```python
from build123d import *

# Parameters (mm, degrees)
SKETCH1_W                                       = 200
SKETCH1_H                                       = 320
BOSS_EXTRUDE1_DEPTH                             = 3.175
CSK_FOR_M3_FLAT_HEAD_MACHINE_SCREW1_D           = 3.4
CSK_FOR_M3_FLAT_HEAD_MACHINE_SCREW1_CSINK_D     = 6.3
CSK_FOR_M3_FLAT_HEAD_MACHINE_SCREW1_CSINK_ANGLE = 90
MIRROR2_COPY_1_D                                = 3.4
MIRROR2_COPY_1_CSINK_D                          = 6.3
MIRROR2_COPY_1_CSINK_ANGLE                      = 90
CSK_FOR_M4_FLAT_HEAD_MACHINE_SCREW1_AT_2_COUNT  = 2
CSK_FOR_M4_FLAT_HEAD_MACHINE_SCREW1_AT_2_PITCH  = 64.709214954
CSK_FOR_M4_FLAT_HEAD_MACHINE_SCREW1_AT_3_COUNT  = 2
CSK_FOR_M4_FLAT_HEAD_MACHINE_SCREW1_AT_3_PITCH  = 44.433123905
CSK_FOR_M4_FLAT_HEAD_MACHINE_SCREW1_AT_4_COUNT  = 2
CSK_FOR_M4_FLAT_HEAD_MACHINE_SCREW1_AT_4_PITCH  = 75.973301231
CSK_FOR_M4_FLAT_HEAD_MACHINE_SCREW1_AT_5_COUNT  = 2
CSK_FOR_M4_FLAT_HEAD_MACHINE_SCREW1_AT_5_PITCH  = 78.545162168
CSK_FOR_M4_FLAT_HEAD_MACHINE_SCREW1_AT_6_COUNT  = 2
CSK_FOR_M4_FLAT_HEAD_MACHINE_SCREW1_AT_6_PITCH  = 60.96
CSK_FOR_M4_FLAT_HEAD_MACHINE_SCREW1_AT_7_COUNT  = 2
CSK_FOR_M4_FLAT_HEAD_MACHINE_SCREW1_AT_7_PITCH  = 49.53
CSK_FOR_M4_FLAT_HEAD_MACHINE_SCREW1_AT_8_COUNT  = 2
CSK_FOR_M4_FLAT_HEAD_MACHINE_SCREW1_AT_8_PITCH  = 89.358393562
CSK_FOR_M4_FLAT_HEAD_MACHINE_SCREW1_AT_9_COUNT  = 2
CSK_FOR_M4_FLAT_HEAD_MACHINE_SCREW1_AT_9_PITCH  = 245.539452023
CSK_FOR_M4_FLAT_HEAD_MACHINE_SCREW1_AT_1_COUNT  = 2
CSK_FOR_M4_FLAT_HEAD_MACHINE_SCREW1_AT_1_PITCH  = 233.172012257
CSK_FOR_M4_FLAT_HEAD_MACHINE_SCREW1_2_COUNT     = 2
CSK_FOR_M4_FLAT_HEAD_MACHINE_SCREW1_2_PITCH     = 183.831254144
CSK_FOR_M4_FLAT_HEAD_MACHINE_SCREW1_3_COUNT     = 2
CSK_FOR_M4_FLAT_HEAD_MACHINE_SCREW1_3_PITCH     = 199.284633627
CSK_FOR_M4_FLAT_HEAD_MACHINE_SCREW1_4_COUNT     = 2
CSK_FOR_M4_FLAT_HEAD_MACHINE_SCREW1_4_PITCH     = 64.860029294
CSK_FOR_M4_FLAT_HEAD_MACHINE_SCREW1_5_COUNT     = 2
CSK_FOR_M4_FLAT_HEAD_MACHINE_SCREW1_5_PITCH     = 190.701291553
CSK_FOR_M4_FLAT_HEAD_MACHINE_SCREW1_6_COUNT     = 2
CSK_FOR_M4_FLAT_HEAD_MACHINE_SCREW1_6_PITCH     = 183.209354019
CSK_FOR_M4_FLAT_HEAD_MACHINE_SCREW1_7_COUNT     = 2
CSK_FOR_M4_FLAT_HEAD_MACHINE_SCREW1_7_PITCH     = 69.556924889
SKETCH8_R                                       = 19
CUT_EXTRUDE1_DEPTH                              = 4.175


with BuildPart() as part:
    # Sketch1 → Boss-Extrude1 (new body)
    with BuildSketch(Plane(origin=(0, 0, 0), x_dir=(1, 0, 0), z_dir=(0, 1, 0))):
        Rectangle(SKETCH1_W, SKETCH1_H)
    extrude(amount=BOSS_EXTRUDE1_DEPTH)

    # CSK for M3 Flat Head Machine Screw1 (through all)
    with Locations(Plane.XZ):
        with Locations((-95, 155), (-85, 155), (-95, 145), (-95, 135), (-95, 105), (-95, 95)):
            csk_for_m3_flat_head_machine_screw1 = CounterSinkHole(CSK_FOR_M3_FLAT_HEAD_MACHINE_SCREW1_D / 2, CSK_FOR_M3_FLAT_HEAD_MACHINE_SCREW1_CSINK_D / 2, counter_sink_angle=CSK_FOR_M3_FLAT_HEAD_MACHINE_SCREW1_CSINK_ANGLE)

    # Mirror1: CSK for M3 Flat Head Machine Screw1 across plane
    add(csk_for_m3_flat_head_machine_screw1.mirror(Plane(origin=(0, 0, 0), x_dir=(0, 0, 1), z_dir=(1, 0, 0))), mode=Mode.SUBTRACT)

    # Mirror2: CSK for M3 Flat Head Machine Screw1 across plane
    add(csk_for_m3_flat_head_machine_screw1.mirror(Plane.XY), mode=Mode.SUBTRACT)

    # Mirror2 copy 1 (through all)
    with Locations(Plane(origin=(0, 0, 0), x_dir=(-1, 0, 0), z_dir=(0, -1, 0))):
        with Locations((-95, 155), (-85, 155), (-95, 145), (-95, 135), (-95, 105), (-95, 95)):
            CounterSinkHole(MIRROR2_COPY_1_D / 2, MIRROR2_COPY_1_CSINK_D / 2, counter_sink_angle=MIRROR2_COPY_1_CSINK_ANGLE)

    # Sketch6 → CSK for M4 Flat Head Machine Screw1 (revolve, cut)
    with BuildSketch(Plane(origin=(-9.04, 0, 91.47), x_dir=(0, 0, -1), z_dir=(1, 0, 0))):
        Polygon((0, 0), (0, 3.175), (2.25, 3.175), (2.25, 2.45), (4.7, 0), align=None)
    csk_for_m4_flat_head_machine_screw1 = revolve(axis=Axis((-9.04, -6.35, 91.47), (0, 1, 0)), mode=Mode.SUBTRACT)

    # CSK for M4 Flat Head Machine Screw1 at 2: CSK for M4 Flat Head Machine Screw1 ×2
    with Locations(*[Vector(0.634221881, 0, 0.773151089) * (i * CSK_FOR_M4_FLAT_HEAD_MACHINE_SCREW1_AT_2_PITCH) for i in range(1, CSK_FOR_M4_FLAT_HEAD_MACHINE_SCREW1_AT_2_COUNT)]):
        add(csk_for_m4_flat_head_machine_screw1, mode=Mode.SUBTRACT)

    # CSK for M4 Flat Head Machine Screw1 at 3: CSK for M4 Flat Head Machine Screw1 ×2
    with Locations(*[Vector(0.923635261, 0, 0.383272624) * (i * CSK_FOR_M4_FLAT_HEAD_MACHINE_SCREW1_AT_3_PITCH) for i in range(1, CSK_FOR_M4_FLAT_HEAD_MACHINE_SCREW1_AT_3_COUNT)]):
        add(csk_for_m4_flat_head_machine_screw1, mode=Mode.SUBTRACT)

    # CSK for M4 Flat Head Machine Screw1 at 4: CSK for M4 Flat Head Machine Screw1 ×2
    with Locations(*[Vector(0.974552886, 0, 0.224157694) * (i * CSK_FOR_M4_FLAT_HEAD_MACHINE_SCREW1_AT_4_PITCH) for i in range(1, CSK_FOR_M4_FLAT_HEAD_MACHINE_SCREW1_AT_4_COUNT)]):
        add(csk_for_m4_flat_head_machine_screw1, mode=Mode.SUBTRACT)

    # CSK for M4 Flat Head Machine Screw1 at 5: CSK for M4 Flat Head Machine Screw1 ×2
    with Locations(*[Vector(-0.776114, 0, 0.630592625) * (i * CSK_FOR_M4_FLAT_HEAD_MACHINE_SCREW1_AT_5_PITCH) for i in range(1, CSK_FOR_M4_FLAT_HEAD_MACHINE_SCREW1_AT_5_COUNT)]):
        add(csk_for_m4_flat_head_machine_screw1, mode=Mode.SUBTRACT)

    # CSK for M4 Flat Head Machine Screw1 at 6: CSK for M4 Flat Head Machine Screw1 ×2
    with Locations(*[(-i * CSK_FOR_M4_FLAT_HEAD_MACHINE_SCREW1_AT_6_PITCH, 0, 0) for i in range(1, CSK_FOR_M4_FLAT_HEAD_MACHINE_SCREW1_AT_6_COUNT)]):
        add(csk_for_m4_flat_head_machine_screw1, mode=Mode.SUBTRACT)

    # CSK for M4 Flat Head Machine Screw1 at 7: CSK for M4 Flat Head Machine Screw1 ×2
    with Locations(*[(0, 0, i * CSK_FOR_M4_FLAT_HEAD_MACHINE_SCREW1_AT_7_PITCH) for i in range(1, CSK_FOR_M4_FLAT_HEAD_MACHINE_SCREW1_AT_7_COUNT)]):
        add(csk_for_m4_flat_head_machine_screw1, mode=Mode.SUBTRACT)

    # CSK for M4 Flat Head Machine Screw1 at 8: CSK for M4 Flat Head Machine Screw1 ×2
    with Locations(*[Vector(0.828573535, 0, 0.559880253) * (i * CSK_FOR_M4_FLAT_HEAD_MACHINE_SCREW1_AT_8_PITCH) for i in range(1, CSK_FOR_M4_FLAT_HEAD_MACHINE_SCREW1_AT_8_COUNT)]):
        add(csk_for_m4_flat_head_machine_screw1, mode=Mode.SUBTRACT)

    # CSK for M4 Flat Head Machine Screw1 at 9: CSK for M4 Flat Head Machine Screw1 ×2
    with Locations(*[Vector(0.321903463, 0, -0.946772497) * (i * CSK_FOR_M4_FLAT_HEAD_MACHINE_SCREW1_AT_9_PITCH) for i in range(1, CSK_FOR_M4_FLAT_HEAD_MACHINE_SCREW1_AT_9_COUNT)]):
        add(csk_for_m4_flat_head_machine_screw1, mode=Mode.SUBTRACT)

    # CSK for M4 Flat Head Machine Screw1 at 1: CSK for M4 Flat Head Machine Screw1 ×2
    with Locations(*[Vector(0.077539323, 0, -0.996989295) * (i * CSK_FOR_M4_FLAT_HEAD_MACHINE_SCREW1_AT_1_PITCH) for i in range(1, CSK_FOR_M4_FLAT_HEAD_MACHINE_SCREW1_AT_1_COUNT)]):
        add(csk_for_m4_flat_head_machine_screw1, mode=Mode.SUBTRACT)

    # CSK for M4 Flat Head Machine Screw1  2: CSK for M4 Flat Head Machine Screw1 ×2
    with Locations(*[Vector(0.098351067, 0, -0.995151781) * (i * CSK_FOR_M4_FLAT_HEAD_MACHINE_SCREW1_2_PITCH) for i in range(1, CSK_FOR_M4_FLAT_HEAD_MACHINE_SCREW1_2_COUNT)]):
        add(csk_for_m4_flat_head_machine_screw1, mode=Mode.SUBTRACT)

    # CSK for M4 Flat Head Machine Screw1  3: CSK for M4 Flat Head Machine Screw1 ×2
    with Locations(*[Vector(0.396618638, 0, -0.917983473) * (i * CSK_FOR_M4_FLAT_HEAD_MACHINE_SCREW1_3_PITCH) for i in range(1, CSK_FOR_M4_FLAT_HEAD_MACHINE_SCREW1_3_COUNT)]):
        add(csk_for_m4_flat_head_machine_screw1, mode=Mode.SUBTRACT)

    # CSK for M4 Flat Head Machine Screw1  4: CSK for M4 Flat Head Machine Screw1 ×2
    with Locations(*[Vector(0.981343991, 0, -0.192260166) * (i * CSK_FOR_M4_FLAT_HEAD_MACHINE_SCREW1_4_PITCH) for i in range(1, CSK_FOR_M4_FLAT_HEAD_MACHINE_SCREW1_4_COUNT)]):
        add(csk_for_m4_flat_head_machine_screw1, mode=Mode.SUBTRACT)

    # CSK for M4 Flat Head Machine Screw1  5: CSK for M4 Flat Head Machine Screw1 ×2
    with Locations(*[Vector(0.453641395, 0, -0.891184316) * (i * CSK_FOR_M4_FLAT_HEAD_MACHINE_SCREW1_5_PITCH) for i in range(1, CSK_FOR_M4_FLAT_HEAD_MACHINE_SCREW1_5_COUNT)]):
        add(csk_for_m4_flat_head_machine_screw1, mode=Mode.SUBTRACT)

    # CSK for M4 Flat Head Machine Screw1  6: CSK for M4 Flat Head Machine Screw1 ×2
    with Locations(*[Vector(-0.37350713, 0, -0.927627309) * (i * CSK_FOR_M4_FLAT_HEAD_MACHINE_SCREW1_6_PITCH) for i in range(1, CSK_FOR_M4_FLAT_HEAD_MACHINE_SCREW1_6_COUNT)]):
        add(csk_for_m4_flat_head_machine_screw1, mode=Mode.SUBTRACT)

    # CSK for M4 Flat Head Machine Screw1  7: CSK for M4 Flat Head Machine Screw1 ×2
    with Locations(*[Vector(-0.983798523, 0, -0.179277621) * (i * CSK_FOR_M4_FLAT_HEAD_MACHINE_SCREW1_7_PITCH) for i in range(1, CSK_FOR_M4_FLAT_HEAD_MACHINE_SCREW1_7_COUNT)]):
        add(csk_for_m4_flat_head_machine_screw1, mode=Mode.SUBTRACT)

    # Sketch8 → Cut-Extrude1 (cut, through all)
    with BuildSketch(Plane(origin=(0, 3.175, 0), x_dir=(1, 0, 0), z_dir=(0, 1, 0))):
        with Locations((48.5, -125)):
            Circle(SKETCH8_R)
    extrude(amount=-CUT_EXTRUDE1_DEPTH, mode=Mode.SUBTRACT)


solid = part.part
```
Source: CAD feature listing. Evaluate the final solid. Frame: model axes, mm. Coordinates: 2 decimals unless noted, no trailing zeros. Loops run counter-clockwise (first coordinate to the right, second up) from the corner with the lowest first, then second, coordinate; pieces in that order, holes last. Notation, with made-up numbers: M 62.5,-35.75 L 79.5,-35.75 A25 ccw 79.5,2.25 Z; hole C 2,56.5 d1. An arc over 180 degrees is marked long. Use a Markdown table: item, result. Add a question column.
Q1. Draft query along X for faces 1 (the conical face through (11.386, 2.297, -90.949)), 2 (the flat face through (-1, 0, -2)). Return one class per face: pulls with the +X half, pulls with the -X half, needs draft (parallel to the pull), parting line crosses it, or undercut.
Q2. Section query A-A, the plane z = 125. Return loops of the section in (x, y) (3 decimals).
Q3. Section query B-B, the plane x = 42. Return loops of the section in (y, z) (3 decimals).
Q4. Section query C-C, the plane y = 0.85. State how many separate pieces and enclosed holes the cut face has, and give its area (3 significant figures).
Q5. First-contact query: pin 1 (2.5 mm diameter, centred on x = 70, z = -91.47, fed in from +Y); pin 2 (4 mm diameter, centred on x = 85, z = -155, fed in from -Y); pin 3 (7 mm diameter, centred on x = -77.47, z = -78.48, fed in from -Y); pin 4 (5.5 mm diameter, centred on x = -95, z = -95, fed in from -Y). Flat tips, straight axial feed; report the tip coordinate or a pass-through.
Q6. Material intervals for L1, parallel to X at y = 2.75, z = -91.47; L2, parallel to X at y = 2.4, z = -105; L3, parallel to X at y = 0.95, z = -144, sorted ascending.
Result:
| question | item | result |
|---|---|---|
| 1 | face 1 | undercut |
| 1 | face 2 | needs draft |
| 2 | outline | M -100,0 L 29.5,0 L 29.5,3.175 L -100,3.175 Z; M 67.5,0 L 100,0 L 100,3.175 L 67.5,3.175 Z |
| 3 | outline | M 0,-160 L 3.175,-160 L 3.175,107.146 L 0,107.146 Z; M 0,142.854 L 3.175,142.854 L 3.175,160 L 0,160 Z |
| 4 | separate pieces | 1 |
| 4 | enclosed holes | 41 |
| 4 | area | 61,700 mm2 |
| 5 | pin 1 | passes through |
| 5 | pin 2 | stops at y = 1.15 |
| 5 | pin 3 | stops at y = 1.2 |
| 5 | pin 4 | stops at y = 0.4 |
| 6 | L1 | x = -100 to 6.79, 11.29 to 67.75, 72.25 to 100 |
| 6 | L2 | x = -100 to -96.7, -93.3 to 93.3, 96.7 to 100 |
| 6 | L3 | x = -100 to -96.96, -93.04 to 6.79, 11.29 to 67.75, 72.25 to 93.04, 96.96 to 100 |
